Input: part model. Units: mm. Frame: model coordinates. Give positions to 0.01 mm unless a question says otherwise; leave off trailing zeros. Loops run counter-clockwise (first coordinate to the right, second up) from the corner with the lowest first, then second, coordinate; pieces in that order, holes last. Notation, with made-up numbers: M 34.25,50 L 45.25,50 A19 ccw 45.25,68 Z; hole C 69,3 d3. An arc over 180 degrees is marked long. One line per item, written item: value. Start each with the question number.
(1) Section A-A on x = 3. Output: boundary loops of the cut face in (y, z), plus the area to 3 significant figures.
(2) Ray query, line 1 along Z through (x, y) = (19, -0.25); line 2 along Y through (x, z) = (2, -1.95); line 3 along Y through (x, z) = (-12, 1.9). Return the intervals inside material, ascending. Write a range as from..to.
(3) Pin query (flat end, axial travel): P1, Ø2, axis at x = 0.5, z = -2, coming from the +Y side; P2, Ø3, axis at x = 15.5, z = 2, coming from the -Y side; P3, Ø1.5, axis at x = 1, y = -1, coming from the -Z side. Return the tip coordinate at first contact, or that it passes through.
(4) Section B-B on x = 15.5. Output: boundary loops of the cut face in (y, z).
```python
from build123d import *

# Parameters (mm, degrees)
SKETCH2_R                     = 2.5
BOSS_EXTRUDE1_DEPTH           = 21
BOSS_EXTRUDE1_TAPER           = 1.15
BOSS_EXTRUDE1_OTHER_WAY_DEPTH = 21
BOSS_EXTRUDE1_OTHER_WAY_TAPER = -1.15


with BuildPart() as part:
    # Sketch2 → Boss-Extrude1 (new body)
    with BuildSketch(Plane(origin=(0, 0, 0), x_dir=(0, 0, -1), z_dir=(1, 0, 0))):
        Circle(SKETCH2_R)
    extrude(amount=BOSS_EXTRUDE1_DEPTH, taper=BOSS_EXTRUDE1_TAPER)

    # Sketch2 → Boss-Extrude1 other way (add)
    with BuildSketch(Plane(origin=(0, 0, 0), x_dir=(0, 0, -1), z_dir=(1, 0, 0))):
        Circle(SKETCH2_R)
    extrude(amount=-BOSS_EXTRUDE1_OTHER_WAY_DEPTH, taper=BOSS_EXTRUDE1_OTHER_WAY_TAPER)

    # Fillet1
    # an asymmetric fillet: 2.8, 1 mm, written as the material it takes off along each edge
    with BuildSketch(Plane(origin=(-21, 0, 0), x_dir=(0, 0, -1), z_dir=(0, -1, 0))) as fillet1_piece_1:
        with BuildLine():
            Bezier((2.900351568, 1.056195829), (2.921553624, 0), (0.100915548, 0), weights=[1, 0.699975021, 1])
            Line((0.100915548, 0), (2.921553624, 0))
            Line((2.921553624, 0), (2.900351568, 1.056195829))
        make_face()
    revolve(axis=Axis((-21, 0, 0), (1, 0, 0)), mode=Mode.SUBTRACT)

    # Fillet2
    # an asymmetric fillet: 2, 1 mm, written as the material it takes off along each edge
    with BuildSketch(Plane(origin=(21, 0, 0), x_dir=(0, 0, -1), z_dir=(0, 1, 0))) as fillet2_piece_1:
        with BuildLine():
            Bezier((2.097714591, 0.959860122), (2.078446376, 0), (0.098117434, 0), weights=[1, 0.714167326, 1])
            Line((0.098117434, 0), (2.078446376, 0))
            Line((2.078446376, 0), (2.097714591, 0.959860122))
        make_face()
    revolve(axis=Axis((21, 0, 0), (-1, 0, 0)), mode=Mode.SUBTRACT)


solid = part.part
```
Output values:
1. outline: C 0,0 d4.88
1. area: 18.7 mm²
2. line 1: z = -2.1..2.1
2. line 2: y = -1.5..1.5
2. line 3: y = -1.98..1.98
3. P1: stops at y = 2.28
3. P2: stops at y = -2.13
3. P3: stops at z = -2.47
4. outline: C 0,0 d4.38
